Here's how the part is built. I have some questions about the finished solid (model axes, mm). A direction names the side the tool comes from. Give positions to 0.01 mm unless a question says otherwise; leave off trailing zeros. Order: outer loops, then holes, each group sorted by start corner. A loop starts at its lowest first (then second) coordinate and runs counter-clockwise, first axis right, second up. Notation, with made-up numbers: (-3, 16) -> (11, 16) arc R23 ccw to (11, 52) -> close; hole circle Ø11 at (53, 79.25). An arc over 180 degrees is marked (long way). Write each question's results on one line, items separated by ' | '. Start each with the question number.
Q1. Imagine slicing it at C-C, the plane z = 5.5. Please give me the cut outline in (x, y).
Q2. For faces 4 (the face through (-3.89, -7, -27)), 5 (the face through (0, 0, 0)), 6 (the face through (-4, -5.45, 8)), which set-ups out of +Z, -Z, +X, -X, +Y, -Y let a thin tool reach every point of the face, with its end or its side?
Q3. Imagine slicing it at D-D, the plane y = -4.95. Please give me the cut outline in (x, z).
Q4. Imagine slicing it at B-B, the plane y = 5.05. Please give me the cut outline in (x, z), then the cut area to 3 significant figures.
Q5. Thinking about a two-plate mould opening in Z: for faces 1 (the face through (5.71, -3.94, 1.48)), 2 (the face through (0, 0, -19.25)), 3 (the face through (0, 3, -22.25)), which applies, pulls with the +Z half, pulls with the -Z half, needs draft (parallel to the pull), parting line crosses it, or undercut?
Q6. Imagine slicing it at A-A, the plane y = -2.25. Please give me the cut outline in (x, z), then the cut area to 3 significant figures.
Q7. I need wall thicknesses on line 1 along X through (y, z) = (-6.1, 8.5); line 2 along Z through (x, y) = (8.25, -3.5); line 3 along Z through (x, y) = (-3.5, -6). Which ranges of each line are inside material? Lowest first, please. Write a range as [from, to].
Q8. I'm going to push flat-ended pins straight in: pin 1 (3.5 mm diameter, centred on x = -1, z = 8, fed in from +Y); pin 2 (2.5 mm diameter, centred on x = 5.17, y = 5.05, fed in from -Z); pin 3 (9.5 mm diameter, centred on x = 3.5, y = -0.5, fed in from +Z); pin 4 (4 mm diameter, centred on x = 6, z = 6, fed in from +Y). Where does each tip first touch, or does it pass through?
```python
from build123d import *

# Parameters (mm, degrees)
SKETCH1_W             = 22.22
SKETCH1_H             = 15.9
SKETCH1_R             = 1.5
BOSS_EXTRUDE1_DEPTH   = 3
SKETCH3_W             = 9
SKETCH3_H             = 2.5
BOSS_EXTRUDE2_DEPTH   = 15
FILLET2_R             = 2
CUT_EXTRUDE1_REACH    = 4.5
SKETCH5_R             = 1.75
LPATTERN2_COUNT       = 2
LPATTERN2_PITCH       = 6.95
BODY_MOVE_COPY3_ANGLE = 180
SKETCH11_W            = 22.249975
SKETCH11_H            = 3
BOSS_EXTRUDE3_DEPTH   = 22.22
SKETCH12_W            = 3
SKETCH12_H            = 3
BOSS_EXTRUDE4_DEPTH   = 22.22


with BuildPart() as part:
    # Sketch1 → Boss-Extrude1 (new body)
    with BuildSketch(Plane.XY):
        Rectangle(SKETCH1_W, SKETCH1_H)
        with Locations((-5.17, 5.05)):
            Circle(SKETCH1_R, mode=Mode.SUBTRACT)
        with Locations((6.82, -4.95)):
            Circle(SKETCH1_R, mode=Mode.SUBTRACT)
    extrude(amount=BOSS_EXTRUDE1_DEPTH)

    # Sketch3 → Boss-Extrude2 (add)
    with BuildSketch(Plane.ZY.offset(11.11)):
        with Locations((7.5, -6.7)):
            Rectangle(SKETCH3_W, SKETCH3_H)
    extrude(amount=-BOSS_EXTRUDE2_DEPTH)

    # Fillet2
    fillet2_edges = [part.edges().sort_by_distance(p)[0] for p in [
        (-3.61, -5.45, 3),
    ]]
    fillet(fillet2_edges, radius=FILLET2_R)

    # Sketch5 → Cut-Extrude1 (cut, up to next)
    with BuildSketch(Plane(origin=(0, -5.45, 0), x_dir=(1, 0, 0), z_dir=(0, 1, 0)), mode=Mode.PRIVATE) as cut_extrude1_sk1:
        with Locations((-8.11, -8.5)):
            Circle(SKETCH5_R)
    cut_extrude1_tool1 = extrude(cut_extrude1_sk1.sketch, amount=-CUT_EXTRUDE1_REACH, mode=Mode.PRIVATE) & part.part
    add(cut_extrude1_tool1.solids().sort_by_distance((-8.11, -5.45, 8.5))[0], mode=Mode.SUBTRACT)
    # Sketch5 → Cut-Extrude1 (cut, up to next)
    with BuildSketch(Plane(origin=(0, -5.45, 0), x_dir=(1, 0, 0), z_dir=(0, 1, 0)), mode=Mode.PRIVATE) as cut_extrude1_sk2:
        with Locations((0.89, -8.5)):
            Circle(SKETCH5_R)
    cut_extrude1_tool2 = extrude(cut_extrude1_sk2.sketch, amount=-CUT_EXTRUDE1_REACH, mode=Mode.PRIVATE) & part.part
    add(cut_extrude1_tool2.solids().sort_by_distance((0.89, -5.45, 8.5))[0], mode=Mode.SUBTRACT)


with BuildPart() as lpattern2_1:
    # LPattern2: pattern copy
    add(part.part.moved(Location(Vector(0, 0, -1) * (1 * LPATTERN2_PITCH))))


with BuildPart() as lpattern2_1_1:
    # Body-Move/Copy3: moved
    add(lpattern2_1.part.rotate(Axis((1.25e-05, 0, -13.0999875), (0, 1, 0)), BODY_MOVE_COPY3_ANGLE))

    # Sketch11 → Boss-Extrude3 (add)
    with BuildSketch(Plane.ZY.offset(11.109975)):
        with Locations((-11.1249875, 9.45)):
            Rectangle(SKETCH11_W, SKETCH11_H)
    extrude(amount=-BOSS_EXTRUDE3_DEPTH)


with BuildPart() as part_1:
    add(part.part)

    add(lpattern2_1_1.part)  # Boss-Extrude4 merges LPattern2_1
    # Sketch12 → Boss-Extrude4 (add)
    with BuildSketch(Plane.ZY.offset(11.109975)):
        with Locations((1.5, 9.45)):
            Rectangle(SKETCH12_W, SKETCH12_H)
    extrude(amount=-BOSS_EXTRUDE4_DEPTH)


solid = part_1.part
```
Geometry check:
1) outline: (-11.11, -7.95) -> (3.89, -7.95) -> (3.89, -5.45) -> (-11.11, -5.45) -> close
2) face 4: -Z, -X, +Y, -Y | face 5: +X, -X, -Y | face 6: +Z, +X, -X, +Y
3) outline: (-11.11, -22.25) -> (-8.32, -22.25) -> (-8.32, -19.25) -> (-11.11, -19.25) -> close; (-11.11, 0) -> (5.32, 0) -> (5.32, 3) -> (3.89, 3) -> (3.89, 3.68) -> (-11.11, 3.68) -> close; (-5.32, -22.25) -> (-3.89, -22.25) -> (-3.89, -22.93) -> (11.11, -22.93) -> (11.11, -19.25) -> (-5.32, -19.25) -> close; (8.32, 0) -> (11.11, 0) -> (11.11, 3) -> (8.32, 3) -> close
4) outline: (-11.11, -22.25) -> (3.67, -22.25) -> (3.67, -19.25) -> (-11.11, -19.25) -> close; (-11.11, 0) -> (-6.67, 0) -> (-6.67, 3) -> (-11.11, 3) -> close; (-3.67, 0) -> (11.11, 0) -> (11.11, 3) -> (-3.67, 3) -> close; (6.67, -22.25) -> (11.11, -22.25) -> (11.11, -19.25) -> (6.67, -19.25) -> close | area: 115 mm²
5) face 1: needs draft | face 2: undercut | face 3: pulls with the -Z half
6) outline: (-11.11, -22.25) -> (11.11, -22.25) -> (11.11, -19.25) -> (-11.11, -19.25) -> close; (-11.11, 0) -> (11.11, 0) -> (11.11, 3) -> (-11.11, 3) -> close | area: 133 mm²
7) line 1: [-11.11, -9.86], [-6.36, -0.86], [2.64, 3.89] | line 2: [-22.25, -19.25], [0, 3] | line 3: [-31.25, -19.25], [0, 12]
8) pin 1: y = -5.45 | pin 2: z = 0 | pin 3: z = 4.13 | pin 4: through
